from build123d import *

# Parameters (mm, degrees)
SKETCH002_R  = 28.75
PAD_DEPTH    = 26.5
SKETCH003_R  = 10.5
PAD001_DEPTH = 22


with BuildPart() as part:
    # Sketch → Revolution (revolve)
    with BuildSketch(Plane.XZ):
        with BuildLine():
            Line((-132.5, 0), (0, 0))
            ThreePointArc((0, 0), (-0.319822, 2.215454), (-1.253174, 4.25))
            Line((-1.253174, 4.25), (-2.465385, 4.25))
            Line((-2.465385, 4.25), (-2.465385, 4.75))
            Line((-2.465385, 4.75), (-8.965385, 4.75))
            Line((-8.965385, 4.75), (-8.965385, 4.25))
            Line((-8.965385, 4.25), (-92.465385, 4.25))
            Line((-92.465385, 4.25), (-96.965385, 3.75))
            Line((-96.965385, 3.75), (-96.965385, 2.5))
            Line((-96.965385, 2.5), (-123.5, 2.5))
            Line((-123.5, 2.5), (-123.5, 3))
            Line((-123.5, 3), (-127.5, 3))
            Line((-127.5, 3), (-132.5, 2))
            Line((-132.5, 2), (-132.5, 0))
        make_face()
    revolve(axis=Axis((0, 0, 0), (1, 0, 0)))

    # Sketch002 → Pad (new body)
    with BuildSketch(Plane.XY.offset(-7.5)):
        with Locations((-47.25, 0)):
            Circle(SKETCH002_R)
    extrude(amount=PAD_DEPTH)

    # Sketch003 → Pad001 (join)
    with BuildSketch(Plane.XY.offset(-7.5)):
        with Locations((-47.25, 0)):
            Circle(SKETCH003_R)
    extrude(amount=-PAD001_DEPTH)


solid = part.part
CAD build for the part. Positions are in the model's coordinates, mm. A direction names the side the tool comes from. Round coordinates to 2 decimals unless told otherwise and drop trailing zeros. Write each loop counter-clockwise with the first axis right and the second up, starting at its lowest first coordinate (ties: lowest second). Pieces come first, ordered by that corner, then holes. Notation, with made-up numbers: M 6,76.5 L 10,76.5 A16 cw 10,88.5 Z; hole C 3.25,18 d9. An arc over 180 degrees is marked long. Use a Markdown table: item, result. Add a question column.
1. Slice it at B-B on z = -21. Give the cut face in (x, y).
2. Drill centre lines: probe 1 along Z at (x, y) = (-70.5, 7); probe 2 along X at (y, z) = (-0.5, -27); probe 3 along X at (y, z) = (9, -21.5). Where is each one in solid material? Low to high.
3. Flat gauge pins, fed straight in: P1, Ø5, axis at x = -82, y = 2, coming from the -Z side; P2, Ø5, axis at y = 10.5, z = -15, coming from the -X side; P3, Ø3, axis at y = 2, z = 1, coming from the +X side. Where does each tip first touch, or does it go through?
4. Slice it at A-A on x = -47.25. Give the cut face in (y, z).
5. Slice it at D-D on x = -98.5. Give the cut face in (y, z).
6. Pull direction X, two halves, no side cores. Call faces 4 (the face through (-2.465, 2, 4)), 5 (the face through (-132.5, 0, 0)), 6 (the face through (-13.96, -1.277, 4.054)), 7 (the face through (-96.965, -3, 0)): released by +X, released by -X, zero draft, split by the parting line, or undercut.
7. 3-axis set-ups, long thin cutter, end or side, ignore diameter. For faces 1 (the face through (-57.74, 0.46, -18.35)), 2 (the face through (-8.965, 2, -4)), 3 (the face through (-1.868, -3.584, 2.285)): which of +Z, -Z, +X, -X, +Y, -Y reach the whole face in a straight line?
8. Slice it at C-C on y = 19.5. Give the cut face in (x, z).
Reply:
| question | item | result |
|---|---|---|
| 1 | outline | C -47.25,0 d21 |
| 2 | probe 1 | z = -7.5 to 19 |
| 2 | probe 2 | x = -57.74 to -36.76 |
| 2 | probe 3 | x = -52.66 to -41.84 |
| 3 | P1 | stops at z = -4.25 |
| 3 | P2 | stops at x = -54.05 |
| 3 | P3 | stops at x = -0.03 |
| 4 | outline | M -28.75,-7.5 L -10.5,-7.5 L -10.5,-29.5 L 10.5,-29.5 L 10.5,-7.5 L 28.75,-7.5 L 28.75,19 L -28.75,19 Z |
| 5 | outline | C 0,0 d5 |
| 6 | face 4 | released by +X |
| 6 | face 5 | released by -X |
| 6 | face 6 | undercut |
| 6 | face 7 | undercut |
| 7 | face 1 | -Z |
| 7 | face 2 | none |
| 7 | face 3 | +X |
| 8 | outline | M -68.38,-7.5 L -26.12,-7.5 L -26.12,19 L -68.38,19 Z |
